The model under review builds one solid part; all positions refer to its coordinate system, in mm. Face numbers are marked on the shaded views. Coordinates: 2 decimals unless noted, no trailing zeros. Order: outer loops, then holes, each group sorted by start corner. A loop starts at its lowest first (then second) coordinate and runs counter-clockwise, first axis right, second up.
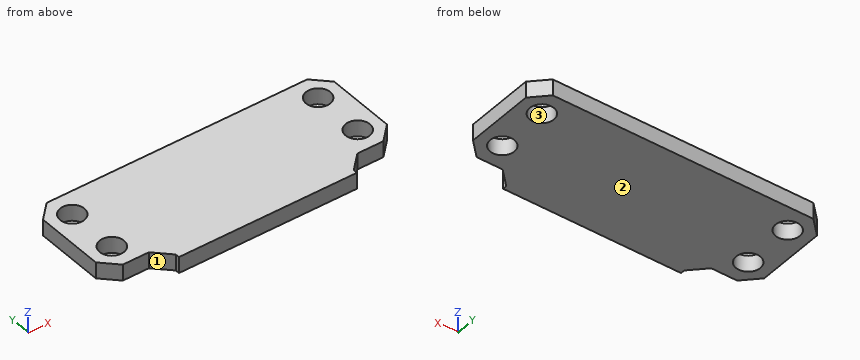
```python
from build123d import *

# Parameters (mm, degrees)
SKETCH1_R           = 3.475
SKETCH1_R_2         = 2.3828
BOSS_EXTRUDE1_DEPTH = 3.175
CHAMFER1_SIZE       = 3
CHAMFER2_SIZE       = 3
SKETCH2_W           = 36.09329734
SKETCH2_H           = 19.05
CUT_EXTRUDE1_DEPTH  = 36.727201556


with BuildPart() as part:
    # Sketch1 → Boss-Extrude1 (new body)
    with BuildSketch(Plane.XY):
        Polygon((17.4625, -21.209), (-17.4625, -21.209), (-17.4625, 1.651), (-28.575, 1.651), (-28.575, 21.209), (28.575, 21.209), (28.575, 1.651), (17.4625, 1.651), align=None)
        with Locations((-9.525, -10.541)):
            Circle(SKETCH1_R, mode=Mode.SUBTRACT)
        with Locations((9.525, -10.541)):
            Circle(SKETCH1_R, mode=Mode.SUBTRACT)
        with Locations((-24.13, 6.35)):
            Circle(SKETCH1_R_2, mode=Mode.SUBTRACT)
        with Locations((-24.13, 16.51)):
            Circle(SKETCH1_R_2, mode=Mode.SUBTRACT)
        with Locations((24.13, 16.51)):
            Circle(SKETCH1_R_2, mode=Mode.SUBTRACT)
        with Locations((24.13, 6.35)):
            Circle(SKETCH1_R_2, mode=Mode.SUBTRACT)
    extrude(amount=BOSS_EXTRUDE1_DEPTH)

    # Chamfer1
    chamfer1_edges = [part.edges().sort_by_distance(p)[0] for p in [
        (-28.575, 1.651, 1.5875),
        (-28.575, 21.209, 1.5875),
        (28.575, 21.209, 1.5875),
        (28.575, 1.651, 1.5875),
    ]]
    chamfer(chamfer1_edges, length=CHAMFER1_SIZE)

    # Chamfer2
    chamfer2_edges = [part.edges().sort_by_distance(p)[0] for p in [
        (17.4625, 1.651, 1.5875),
        (17.4625, -21.209, 1.5875),
        (-17.4625, -21.209, 1.5875),
        (-17.4625, 1.651, 1.5875),
    ]]
    chamfer(chamfer2_edges, length=CHAMFER2_SIZE)

    # Sketch2 → Cut-Extrude1 (cut, through all)
    with BuildSketch(Plane(origin=(0, 0, 0), x_dir=(-1, 0, 0), z_dir=(0, 0, -1))):
        with Locations((0.32904128, -11.684)):
            Rectangle(SKETCH2_W, SKETCH2_H)
    extrude(amount=-CUT_EXTRUDE1_DEPTH, mode=Mode.SUBTRACT)


solid = part.part
```
(1) For pin 1 Ø1 at (x, z) = (22, 1.5) entering from -Y, flat-tipped, find the tip position at first contact; note if it passes through.
A:
pin 1: stops at y = 1.65
(2) We need section C-C, the plane y = 6.35. Write out the cut boundary in (x, z) (3 decimals).
A:
outline: (-28.575, 0) - (-26.513, 0) - (-26.513, 3.175) - (-28.575, 3.175) - close; (-21.747, 0) - (21.747, 0) - (21.747, 3.175) - (-21.747, 3.175) - close; (26.513, 0) - (28.575, 0) - (28.575, 3.175) - (26.513, 3.175) - close
(3) Draft analysis for pull direction X (two halves, no side actions). For the marked faces 1, 2 and 3, state which applies: released by +X, released by -X, zero draft, split by the parting line, or undercut.
A:
face 1: released by -X
face 2: zero draft
face 3: undercut
(4) We need section B-B, the plane x = -24.13. Write out the cut boundary in (y, z) (3 decimals), and give its area (3 significant figures).
A:
outline: (1.651, 0) - (3.967, 0) - (3.967, 3.175) - (1.651, 3.175) - close; (8.733, 0) - (14.127, 0) - (14.127, 3.175) - (8.733, 3.175) - close; (18.893, 0) - (21.209, 0) - (21.209, 3.175) - (18.893, 3.175) - close
area: 31.8 mm2
(5) Wall thickness on probe 1 along Y at (x, z) = (24.13, 0.6); probe 2 along X at (y, z) = (14.5, 0.5) (3 decimals); probe 3 along X at (y, z) = (5.5, 1.6) (3 decimals): over which ranges is each line inside the solid? List them lowest first.
A:
probe 1: y = 1.65 to 3.97, 8.73 to 14.13, 18.89 to 21.21
probe 2: x = -28.575 to -25.41, -22.85 to 22.85, 25.41 to 28.575
probe 3: x = -28.575 to -26.356, -21.904 to 21.904, 26.356 to 28.575
(6) We need section A-A, the plane z = 0.55. Count the separate pieces of the cut face and the enclosed holes in it, and give its area (3 significant figures).
A:
separate pieces: 1
enclosed holes: 4
area: 1,170 mm2
